For this review, take the finished solid that the model builds, in its own axes (mm). A direction names the side the tool comes from. Give positions to 0.01 mm unless a question says otherwise; leave off trailing zeros. Loops run counter-clockwise (first coordinate to the right, second up) from the corner with the lowest first, then second, coordinate; pieces in that order, holes last.
```python
from build123d import *

# Parameters (mm, degrees)
SKETCH_1_R          = 10
EXTRUDE_1_DEPTH     = 24
SKETCH_2_R          = 20
EXTRUDE_2_DEPTH     = 5
M3X0_5_1_D          = 2.5
M3X0_5_1_DEPTH      = 7.5
M3X0_5_1_TIP        = 0.751075774
CUT_EXTRUDE_1_REACH = 42.509
CHAMFER_1_SIZE      = 0.5
CHAMFER_2_SIZE      = 1
CHAMFER_3_SIZE      = 0.5
CHAMFER_4_SIZE      = 2


with BuildPart() as part:
    # 草图1 → 凸台-拉伸1 (new body)
    with BuildSketch(Plane(origin=(0, 0, 0), x_dir=(0, 0, -1), z_dir=(1, 0, 0))):
        Circle(SKETCH_1_R)
        with BuildLine():
            Line((-1.5, 6), (-1.5, 6.5))
            Line((-1.5, 6.5), (1.5, 6.5))
            Line((1.5, 6.5), (1.5, 6))
            Line((1.5, 6), (1.5, 3.708099244))
            ThreePointArc((1.5, 3.708099244), (0, -4), (-1.5, 3.708099244))
            Line((-1.5, 3.708099244), (-1.5, 6))
        make_face(mode=Mode.SUBTRACT)
    extrude(amount=EXTRUDE_1_DEPTH)

    # 草图2 → 凸台-拉伸2 (add)
    with BuildSketch(Plane(origin=(24, 0, 0), x_dir=(0, 0, -1), z_dir=(1, 0, 0))):
        Circle(SKETCH_2_R)
    extrude(amount=EXTRUDE_2_DEPTH)

    # M3x0.5 螺纹孔1
    with Locations(Plane(origin=(29, 0, 0), x_dir=(0, 0, -1), z_dir=(1, 0, 0))):
        with Locations((-13.856406461, 8), (13.856406461, 8), (0, -16)):
            Hole(M3X0_5_1_D / 2, depth=M3X0_5_1_DEPTH)
            with Locations((0, 0, -(M3X0_5_1_DEPTH + M3X0_5_1_TIP / 2))):  # 118° drill point
                Cone(0, M3X0_5_1_D / 2, M3X0_5_1_TIP, mode=Mode.SUBTRACT)

    # 草图5 → 切除-拉伸1 (cut, up to next)
    with BuildSketch(Plane(origin=(29, 0, 0), x_dir=(0, 0, -1), z_dir=(1, 0, 0)), mode=Mode.PRIVATE) as cut_extrude_1_sk1:
        with BuildLine():
            Line((-1.5, 6.5), (-1.5, 3.708099244))
            ThreePointArc((-1.5, 3.708099244), (0, -4), (1.5, 3.708099244))
            Line((1.5, 3.708099244), (1.5, 6.5))
            Line((1.5, 6.5), (-1.5, 6.5))
        make_face()
    cut_extrude_1_tool1 = extrude(cut_extrude_1_sk1.sketch, amount=-CUT_EXTRUDE_1_REACH, mode=Mode.PRIVATE) & part.part
    add(cut_extrude_1_tool1.solids().sort_by_distance((29, 0.697639, 0))[0], mode=Mode.SUBTRACT)

    # 倒角1
    chamfer_1_edges = [part.edges().sort_by_distance(p)[0] for p in [
        (0, -4, 0),
    ]]
    chamfer(chamfer_1_edges, length=CHAMFER_1_SIZE)

    # 倒角2
    chamfer_2_edges = [part.edges().sort_by_distance(p)[0] for p in [
        (0, 0, 10),
    ]]
    chamfer(chamfer_2_edges, length=CHAMFER_2_SIZE)

    # 倒角3
    chamfer_3_edges = [part.edges().sort_by_distance(p)[0] for p in [
        (24, 0, 20),
    ]]
    chamfer(chamfer_3_edges, length=CHAMFER_3_SIZE)

    # 倒角4
    chamfer_4_edges = [part.edges().sort_by_distance(p)[0] for p in [
        (24, 0, 10),
    ]]
    chamfer(chamfer_4_edges, length=CHAMFER_4_SIZE)


solid = part.part
```
Item 1: Take a section at A-A on y = 0. Give the boundary of the cut face in (x, z).
Answer:
outline: (0, -9) - (1, -10) - (22, -10) - (24, -12) - (24, -19.5) - (24.5, -20) - (29, -20) - (29, -4) - (0.5, -4) - (0, -4.5) - close; (0, 4.5) - (0.5, 4) - (29, 4) - (29, 20) - (24.5, 20) - (24, 19.5) - (24, 12) - (22, 10) - (1, 10) - (0, 9) - close
Item 2: Take a section at C-C on z = 0. Give the boundary of the cut face in (x, y).
Answer:
outline: (0, -9) - (1, -10) - (22, -10) - (24, -12) - (24, -14.75) - (29, -14.75) - (29, -4) - (0.5, -4) - (0, -4.5) - close; (0, 6.5) - (29, 6.5) - (29, 20) - (24.5, 20) - (24, 19.5) - (24, 12) - (22, 10) - (1, 10) - (0, 9) - close; (24, -19.5) - (24.5, -20) - (29, -20) - (29, -17.25) - (24, -17.25) - close
Item 3: The part is to be moulded in two halves that separate along Z. For faces 1 (the cylindrical face through (26.718, -19.524, 4.336)), 2 (the flat face through (0, -4, -4)), 3 (the cylindrical face through (26.465, 8.055, 12.608)), say which applies: released by +Z, released by -Z, zero draft, split by the parting line, or undercut.
Answer:
face 1: split by the parting line
face 2: zero draft
face 3: undercut
Item 4: Tool access review of faces 4 (the cylindrical face through (11.35, -9.76, 2.17)), 5 (the flat face through (15, 5, 1.5)), 6 (the flat face through (29, -4.2, 0.3)): name each direction out of +Z, -Z, +X, -X, +Y, -Y from which nothing blocks a thin tool from reaching the whole face with its end or side.
Answer:
face 4: -X
face 5: +X, -X
face 6: +Z, -Z, +X, +Y, -Y
Item 5: Clearance check with flat-ended pins moving along their axes: pin 1 Ø1.5 at (y, z) = (10, -1) entering from -X; pin 2 Ø3 at (x, z) = (17.5, -7.5) entering from -Y; pin 3 Ø4 at (x, y) = (24.5, 15) entering from -Z. State where each tip first meets the part, or that it passes through.
Answer:
pin 1: stops at x = 0.3
pin 2: stops at y = -8
pin 3: stops at z = -15.2
Item 6: Take a section at B-B on x = 27. Give the boundary of the cut face in (y, z), and give its area (3 significant figures).
Answer:
outline: circle Ø40 at (0, 0); hole circle Ø2.5 at (-16, 0); hole (3.71, -1.5) - (6.5, -1.5) - (6.5, 1.5) - (3.71, 1.5) arc R4 ccw (long way) to start; hole circle Ø2.5 at (8, -13.86); hole circle Ø2.5 at (8, 13.86)
area: 1,180 mm2
Item 7: For L1, parallel to Y at x = 27.95, z = 0; L2, parallel to X at y = -13, z = -3; L3, parallel to Z at x = 8.5, y = 3.5, list the stretches that pass through material, from the lowest coordinate up.
Answer:
L1: y = -20 to -17.25, -14.75 to -4, 6.5 to 20
L2: x = 24 to 29
L3: z = -9.37 to -1.94, 1.94 to 9.37
Item 8: Take a section at D-D on x = 23. Give the boundary of the cut face in (y, z), and give its area (3 significant figures).
Answer:
outline: circle Ø22 at (0, 0); hole (3.71, -1.5) - (6.5, -1.5) - (6.5, 1.5) - (3.71, 1.5) arc R4 ccw (long way) to start
area: 322 mm2
